```python
from build123d import *

# Parameters (mm, degrees)
SKIZZE2_W                       = 22
SKIZZE2_H                       = 2.5
SKIZZE2_W_2                     = 24
SKIZZE2_H_2                     = 4
SCHNITT_LINEAR_AUSTRAGEN1_DEPTH = 50
SKIZZE3_R                       = 2.875
SKIZZE3_W                       = 38.5
SKIZZE3_H                       = 7.5
SCHNITT_LINEAR_AUSTRAGEN2_DEPTH = 38.5
FASE1_SIZE                      = 1


with BuildPart() as part:
    # Skizze1 → Rotation1 (revolve)
    with BuildSketch(Plane.XY, mode=Mode.PRIVATE) as rotation1_sk:
        Polygon((0, 0), (0, 8), (-120, 8), (-124.098076211, 9.098076211), (-132, 17), (-132, 20), (-166, 20), (-166, 0), align=None)
    revolve(rotation1_sk.sketch.rotate(Axis((0, 0, 0), (1, 0, 0)), 90), axis=Axis((0, 0, 0), (1, 0, 0)))  # turned: the seam where the file's is

    # Skizze2 → Schnitt-Linear austragen1 (cut, symmetric)
    with BuildSketch(Plane.XY):
        with Locations((-155, 18.75)):
            Rectangle(SKIZZE2_W, SKIZZE2_H)
        with Locations((-154, 0)):
            Rectangle(SKIZZE2_W_2, SKIZZE2_H_2)
        with Locations((-155, -18.75)):
            Rectangle(SKIZZE2_W, SKIZZE2_H)
    extrude(amount=SCHNITT_LINEAR_AUSTRAGEN1_DEPTH, both=True, mode=Mode.SUBTRACT)

    # Skizze3 → Schnitt-Linear austragen2 (cut, through all)
    with BuildSketch(Plane(origin=(0, 17.5, 0), x_dir=(1, 0, 0), z_dir=(0, 1, 0))):
        with Locations(Location((-156.5, 0, 0), (0, 0, 270))):  # turned: the seam where the file's is
            Circle(SKIZZE3_R)
        with Locations((-146.75, -16.25)):
            Rectangle(SKIZZE3_W, SKIZZE3_H)
        with Locations((-146.75, 16.25)):
            Rectangle(SKIZZE3_W, SKIZZE3_H)
    extrude(amount=-SCHNITT_LINEAR_AUSTRAGEN2_DEPTH, mode=Mode.SUBTRACT)

    # Fase1
    fase1_edges = [part.edges().sort_by_distance(p)[0] for p in [
        (0, 0, -8),
    ]]
    chamfer(fase1_edges, length=FASE1_SIZE)


solid = part.part
```
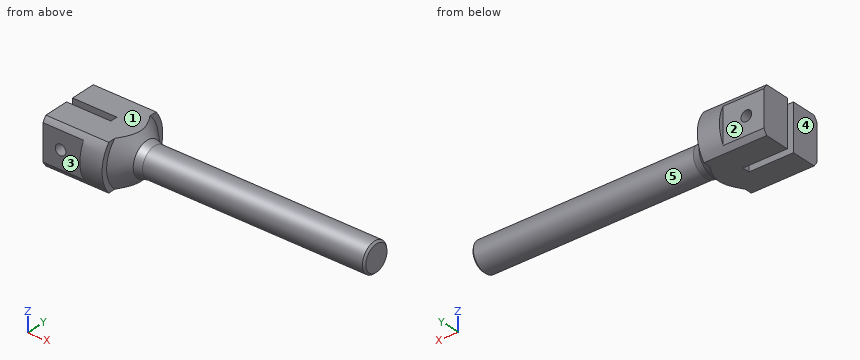
Part model, mm, in its own coordinate system. Face numbers are marked on the shaded views. A direction names the side the tool comes from. Give positions to 0.01 mm unless a question says otherwise; leave off trailing zeros. Write each loop counter-clockwise with the first axis right and the second up, starting at its lowest first coordinate (ties: lowest second). Pieces come first, ordered by that corner, then holes. Notation, with made-up numbers: (88.25, 37) -> (95.25, 37) arc R30 ccw to (95.25, 68) -> close; hole circle Ø2 at (52, 0.5). An arc over 180 degrees is marked (long way). Put each result on its own line as item: value. Start each with the question number.
Item 1: Cut at A-A (z = 0). State how many separate pieces and enclosed holes the cut face has, then the cut area to 3 significant figures.
Item 2: Wall check: L1, parallel to Z at x = -156.5, y = -7.25 (3 decimals); L2, parallel to X at y = 10.5, z = 0 (3 decimals); L3, parallel to Z at x = -156, y = -13. Give the ranges that are in metal, low to high. Write a range as [from, to].
Item 3: Pin check, flat tips, straight feed: pin 1 Ø1.2 at (y, z) = (-19, 2) entering from -X; pin 2 Ø3.5 at (x, z) = (-156.5, 0) entering from -Y; pin 3 Ø7 at (x, z) = (-148, -1.5) entering from -Y; pin 4 Ø8 at (x, y) = (-32, -1) entering from +Z. Stop position of each tip, or through.
Item 4: Cut at D-D (x = -117.5). List the corners of the cut face in (y, z).
Item 5: Cut at B-B (x = -156.5). List the corners of the cut face in (y, z) (1 decimal).
Item 6: Which spindle directions (+Z, -Z, +X, -X, +Y, -Y) get a long thin tool onto all of the face, cutting with end or side? Do the marked faces 1, 2, 3, 4 and 5. Say none if no direction does.
Item 7: Cut at C-C (y = 0). List the corners of the cut face in (x, z), then the cut area to 3 significant figures.
Answer list:
1. separate pieces: 3
1. enclosed holes: 0
1. area: 3,170 mm2
2. L1: z = [-12.5, -2.875], [2.875, 12.5]
2. L2: x = [-166, -159.375], [-153.625, -125.5]
2. L3: z = [-12.5, -2.83], [2.83, 12.5]
3. pin 1: stops at x = -144
3. pin 2: passes through
3. pin 3: stops at y = -17.5
3. pin 4: stops at z = 8
4. outline: circle Ø16 at (0, 0)
5. outline: (-17.5, -9.7) arc R20 ccw to (-15.6, -12.5) -> (-2, -12.5) -> (-2, -2.9) -> (-17.5, -2.9) -> close; (-17.5, 2.9) -> (-2, 2.9) -> (-2, 12.5) -> (-15.6, 12.5) arc R20 ccw to (-17.5, 9.7) -> close; (2, -12.5) -> (15.6, -12.5) arc R20 ccw to (17.5, -9.7) -> (17.5, -2.9) -> (2, -2.9) -> close; (2, 2.9) -> (17.5, 2.9) -> (17.5, 9.7) arc R20 ccw to (15.6, 12.5) -> (2, 12.5) -> close
6. face 1: +Z, +X, -X, +Y, -Y
6. face 2: +Z, -Z, -X, +Y
6. face 3: +Z, -Z, -X, -Y
6. face 4: +Z, -Z, -X, +Y, -Y
6. face 5: +X
7. outline: (-142, -12.5) -> (-127.5, -12.5) -> (-124.1, -9.1) -> (-120, -8) -> (-1, -8) -> (0, -7) -> (0, 7) -> (-1, 8) -> (-120, 8) -> (-124.1, 9.1) -> (-127.5, 12.5) -> (-142, 12.5) -> close
7. area: 2,430 mm2
